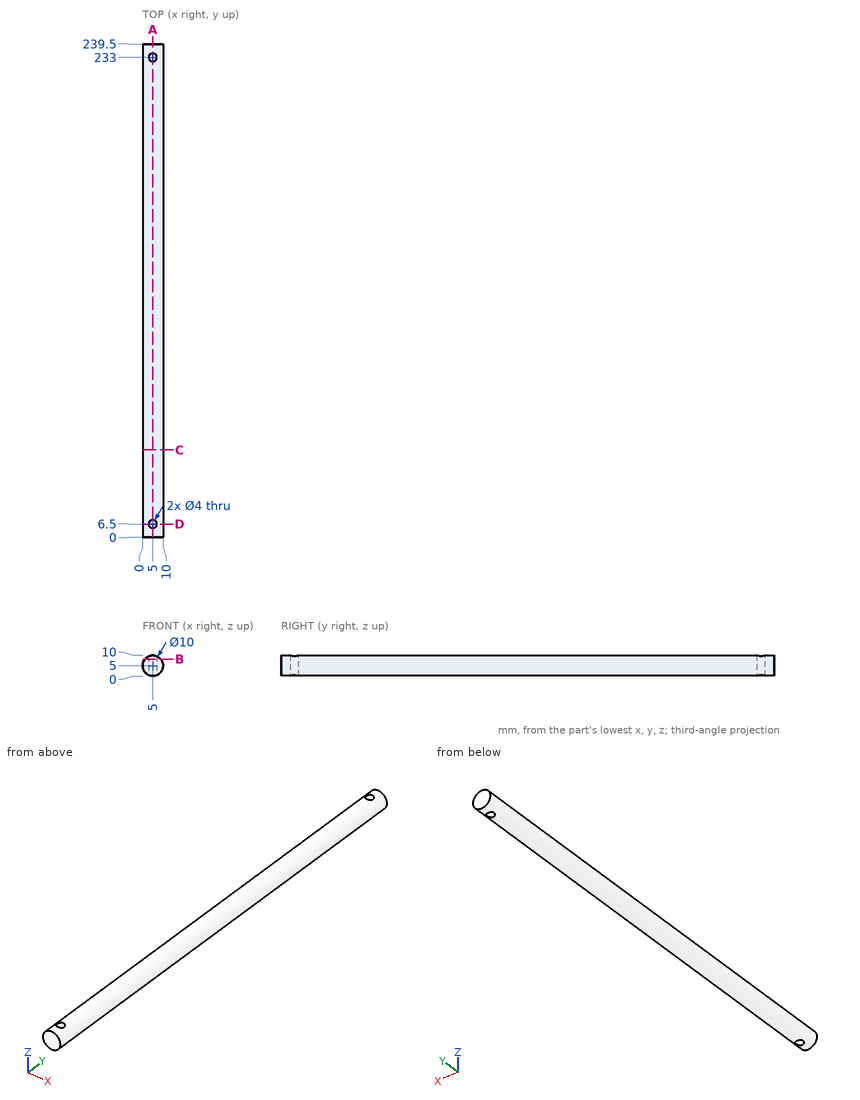
Job drawing, mm, ordinate dimensions from the low corner. One solid piece. Give positions to 0.01 mm unless a question says otherwise; leave off trailing zeros. Write each loop counter-clockwise with the first axis right and the second up, starting at its lowest first coordinate (ties: lowest second). Pieces come first, ordered by that corner, then holes. Notation, with made-up numbers: (-31.5, 26) - (-3.5, 26) arc R19 ccw to (-3.5, 61) - close; hole circle Ø1 at (-33.5, -8.75). An arc over 180 degrees is marked (long way). Answer as CSV lines item,"result".
1. Band-saw the part on D-D (y = 6.5). Write the cut outline in (x, z), and give its area (3 significant figures).
Responses:
outline,"(3, 0.42) - (3, 9.58) arc R5 ccw to start; (7, 0.42) arc R5 ccw to (7, 9.58) - close"
area,"39.6 mm2"
2. Band-saw the part on C-C (y = 42.5). Write the cut outline in (x, z).
Responses:
outline,"circle Ø10 at (5, 5)"
3. Pin check, flat tips, straight feed: pin 1 (1.5 mm diameter, centred on x = 6, y = 99, fed in from -Z); pin 2 (5 mm diameter, centred on y = 50, z = 2, fed in from +X); pin 3 (1.5 mm diameter, centred on x = 7.5, y = 130, fed in from -Z). Stop position of each tip, or through.
Responses:
pin 1,"stops at z = 0.01"
pin 2,"stops at x = 9.97"
pin 3,"stops at z = 0.32"
4. Band-saw the part on A-A (x = 5). Write the cut outline in (y, z).
Responses:
outline,"(0, 0) - (4.5, 0) - (4.5, 10) - (0, 10) - close; (8.5, 0) - (231, 0) - (231, 10) - (8.5, 10) - close; (235, 0) - (239.5, 0) - (239.5, 10) - (235, 10) - close"
5. Band-saw the part on B-B (z = 8.25). Write the cut outline in (x, y).
Responses:
outline,"(1.2, 0) - (8.8, 0) - (8.8, 239.5) - (1.2, 239.5) - close; hole circle Ø4 at (5, 6.5); hole circle Ø4 at (5, 233)"
6. Drill centre lines: L1, parallel to X at y = 6.5, z = 4.5; L2, parallel to Y at x = 4.5, z = 3.5; L3, parallel to Y at x = 4, z = 9. Where is each one in solid material? Low to high. Write a range as [from, to].
Responses:
L1,"x = [0.03, 3], [7, 9.97]"
L2,"y = [0, 4.56], [8.44, 231.06], [234.94, 239.5]"
L3,"y = [0, 4.77], [8.23, 231.27], [234.73, 239.5]"
